The model under review builds one solid part; all positions refer to its coordinate system, in mm. A direction names the side the tool comes from. Round coordinates to 2 decimals unless told otherwise and drop trailing zeros. Use a Markdown table: item, result. Add a question column.
1. Insertion check: P1, Ø6, axis at x = -4, z = 11.5, coming from the -Y side; P2, Ø4, axis at x = 7, z = -32, coming from the -Y side; P3, Ø4, axis at x = 5, z = 13, coming from the +Y side. Each pin has a flat end and moves straight along its axis. Give the tip position at first contact, or say it passes through.
2. To check wall thickness, follow probe 1 along Y at (x, z) = (6, -33.5); probe 2 along Y at (x, z) = (0, -6). State the ranges of each line that lie inside material, in increasing order.
3. The part is to be moulded in two halves that separate along X. For faces 6 (the flat face through (-4, -1.396, -36)), 7 (the cylindrical face through (0.02, -9.05, -10.64)), 8 (the flat face through (1.396, 4, -36)), say which applies: +X half, -X half, draft (parallel to the pull), parting line (faces both ways), or undercut.
4. For faces 1 (the cylindrical face through (0.02, 9.05, 7.89)), 2 (the cylindrical face through (-0.02, 9.05, -10.64)), 3 (the flat face through (-5, -1.396, 9)), 4 (the flat face through (5, 1.396, 9)), 5 (the flat face through (2, 2, -2)), list the 3-axis set-ups (+Z, -Z, +X, -X, +Y, -Y) from which the entire face can be reached by the end or side of a thin tool; tool diameter is ignored.
from build123d import *

# Parameters (mm, degrees)
F0_R      = 9.05
F1_DEPTH  = 17.5
F2_R      = 1.5
F4_DEPTH  = 25
F5_R      = 9.5
F6_DEPTH  = 2
F7_R      = 9.05
F8_DEPTH  = 100
F10_ANGLE = 180
F12_DEPTH = 100.001


with BuildPart() as f1:
    # F0 (on Top) → F1 (new body)
    with BuildSketch(Plane.XY):
        Circle(F0_R)
    extrude(amount=F1_DEPTH)

    # F2
    f2_edges = [f1.edges().sort_by_distance(p)[0] for p in [
        (-9.05, 0, 17.5),
    ]]
    fillet(f2_edges, radius=F2_R)

    # F3 (on face) → F4 (cut)
    with BuildSketch(Plane(origin=(0, 0, 0), x_dir=(1, 0, 0), z_dir=(0, 0, -1))):
        with BuildLine():
            Line((9.05, 0), (9.05, 1.3957661577))
            Line((9.05, 1.3957661577), (8.941718897, 1.3957661577))
            ThreePointArc((8.941718897, 1.3957661577), (9.0228891165, 0.6999799933), (9.05, 0))
        make_face()
        with BuildLine():
            Line((1.3957661577, 8.941718897), (1.3957661577, 9.05))
            Line((1.3957661577, 9.05), (0, 9.05))
            ThreePointArc((0, 9.05), (0.6999799933, 9.0228891165), (1.3957661577, 8.941718897))
        make_face()
        with BuildLine():
            Line((-8.941718897, 1.3957661577), (-9.05, 1.3957661577))
            Line((-9.05, 1.3957661577), (-9.05, 0))
            ThreePointArc((-9.05, 0), (-9.0228891165, 0.6999799933), (-8.941718897, 1.3957661577))
        make_face()
        with BuildLine():
            ThreePointArc((-1.3957661577, 8.941718897), (-0.6999799933, 9.0228891165), (0, 9.05))
            Line((0, 9.05), (-1.3957661577, 9.05))
            Line((-1.3957661577, 9.05), (-1.3957661577, 8.941718897))
        make_face()
        with BuildLine():
            Line((9.05, -1.3957661577), (9.05, 0))
            ThreePointArc((9.05, 0), (9.0228891165, -0.6999799933), (8.941718897, -1.3957661577))
            Line((8.941718897, -1.3957661577), (9.05, -1.3957661577))
        make_face()
        with BuildLine():
            ThreePointArc((-8.941718897, -1.3957661577), (-9.0228891165, -0.6999799933), (-9.05, 0))
            Line((-9.05, 0), (-9.05, -1.3957661577))
            Line((-9.05, -1.3957661577), (-8.941718897, -1.3957661577))
        make_face()
        with BuildLine():
            Line((0, -9.05), (1.3957661577, -9.05))
            Line((1.3957661577, -9.05), (1.3957661577, -8.941718897))
            ThreePointArc((1.3957661577, -8.941718897), (0.6999799933, -9.0228891165), (0, -9.05))
        make_face()
        with BuildLine():
            Line((-1.3957661577, -9.05), (0, -9.05))
            ThreePointArc((0, -9.05), (-0.6999799933, -9.0228891165), (-1.3957661577, -8.941718897))
            Line((-1.3957661577, -8.941718897), (-1.3957661577, -9.05))
        make_face()
        with BuildLine():
            Line((1.3957661577, 1.3957661577), (8.941718897, 1.3957661577))
            ThreePointArc((8.941718897, 1.3957661577), (6.3993163697, 6.3993163697), (1.3957661577, 8.941718897))
            Line((1.3957661577, 8.941718897), (1.3957661577, 1.3957661577))
        make_face()
        with BuildLine():
            ThreePointArc((1.3957661577, -8.941718897), (6.3993163697, -6.3993163697), (8.941718897, -1.3957661577))
            Line((8.941718897, -1.3957661577), (1.3957661577, -1.3957661577))
            Line((1.3957661577, -1.3957661577), (1.3957661577, -8.941718897))
        make_face()
        with BuildLine():
            ThreePointArc((-8.941718897, -1.3957661577), (-6.3993163697, -6.3993163697), (-1.3957661577, -8.941718897))
            Line((-1.3957661577, -8.941718897), (-1.3957661577, -1.3957661577))
            Line((-1.3957661577, -1.3957661577), (-8.941718897, -1.3957661577))
        make_face()
        with BuildLine():
            Line((-1.3957661577, 1.3957661577), (-1.3957661577, 8.941718897))
            ThreePointArc((-1.3957661577, 8.941718897), (-6.3993163697, 6.3993163697), (-8.941718897, 1.3957661577))
            Line((-8.941718897, 1.3957661577), (-1.3957661577, 1.3957661577))
        make_face()
    extrude(amount=-F4_DEPTH, mode=Mode.SUBTRACT)

    # F5 (on face) → F6 (join)
    with BuildSketch(Plane(origin=(0, 0, 0), x_dir=(1, 0, 0), z_dir=(0, 0, -1))):
        Circle(F5_R)
    extrude(amount=F6_DEPTH)

    # F7 (on face) → F8 (join)
    with BuildSketch(Plane(origin=(0, 0, -2), x_dir=(1, 0, 0), z_dir=(0, 0, -1))):
        Circle(F7_R)
    extrude(amount=F8_DEPTH)

    # F9 (on Front) → F10 (revolve, cut)
    with BuildSketch(Plane.XZ):
        with BuildLine():
            Line((-9.05, -19.5278813041), (-9.05, -2))
            ThreePointArc((-9.05, -2), (-9.133446713, -10.7639406521), (-9.05, -19.5278813041))
        make_face()
        with BuildLine():
            Line((9.05, -2), (9.05, -19.5278813041))
            ThreePointArc((9.05, -19.5278813041), (9.133446713, -10.7639406521), (9.05, -2))
        make_face()
        with BuildLine():
            ThreePointArc((9.05, -19.5278813041), (6.38712664, -60.968279359), (0, -102))
            Line((0, -102), (9.05, -102))
            Line((9.05, -102), (9.05, -19.5278813041))
        make_face()
        with BuildLine():
            ThreePointArc((0, -102), (-6.38712664, -60.968279359), (-9.05, -19.5278813041))
            Line((-9.05, -19.5278813041), (-9.05, -102))
            Line((-9.05, -102), (0, -102))
        make_face()
    revolve(axis=Axis((0, 0, -52), (0, 0, -1)), revolution_arc=F10_ANGLE, mode=Mode.SUBTRACT)

    # F11 (on face) → F12 (cut, through all)
    with BuildSketch(Plane(origin=(0, 0, -2), x_dir=(1, 0, 0), z_dir=(0, 0, -1))):
        Polygon((-1.3957661577, -12.4198609713), (-1.3957661577, -7.4198609713), (-1.3957661577, -1.3957661577), (-7.4198609713, -1.3957661577), (-12.4198609713, -1.3957661577), align=None)
        Polygon((-12.4198609713, 1.3957661577), (-7.4198609713, 1.3957661577), (-1.3957661577, 1.3957661577), (-1.3957661577, 7.4198609713), (-1.3957661577, 12.4198609713), align=None)
        Polygon((1.3957661577, 12.4198609713), (1.3957661577, 7.4198609713), (1.3957661577, 1.3957661577), (7.4198609713, 1.3957661577), (12.4198609713, 1.3957661577), align=None)
        Polygon((12.4198609713, -1.3957661577), (7.4198609713, -1.3957661577), (1.3957661577, -1.3957661577), (1.3957661577, -7.4198609713), (1.3957661577, -12.4198609713), align=None)
    extrude(amount=F12_DEPTH, mode=Mode.SUBTRACT)


solid = f1.part
Answer block:
| question | item | result |
|---|---|---|
| 1 | P1 | y = -8.99 |
| 1 | P2 | y = -1.4 |
| 1 | P3 | y = 1.4 |
| 2 | probe 1 | -1.4 to 1.4 |
| 2 | probe 2 | -9.05 to 9.05 |
| 3 | face 6 | draft |
| 3 | face 7 | parting line |
| 3 | face 8 | +X half |
| 4 | face 1 | +Z, +Y |
| 4 | face 2 | -Z, +Y |
| 4 | face 3 | +Z, -X, -Y |
| 4 | face 4 | +Z, +X, +Y |
| 4 | face 5 | -Z |
